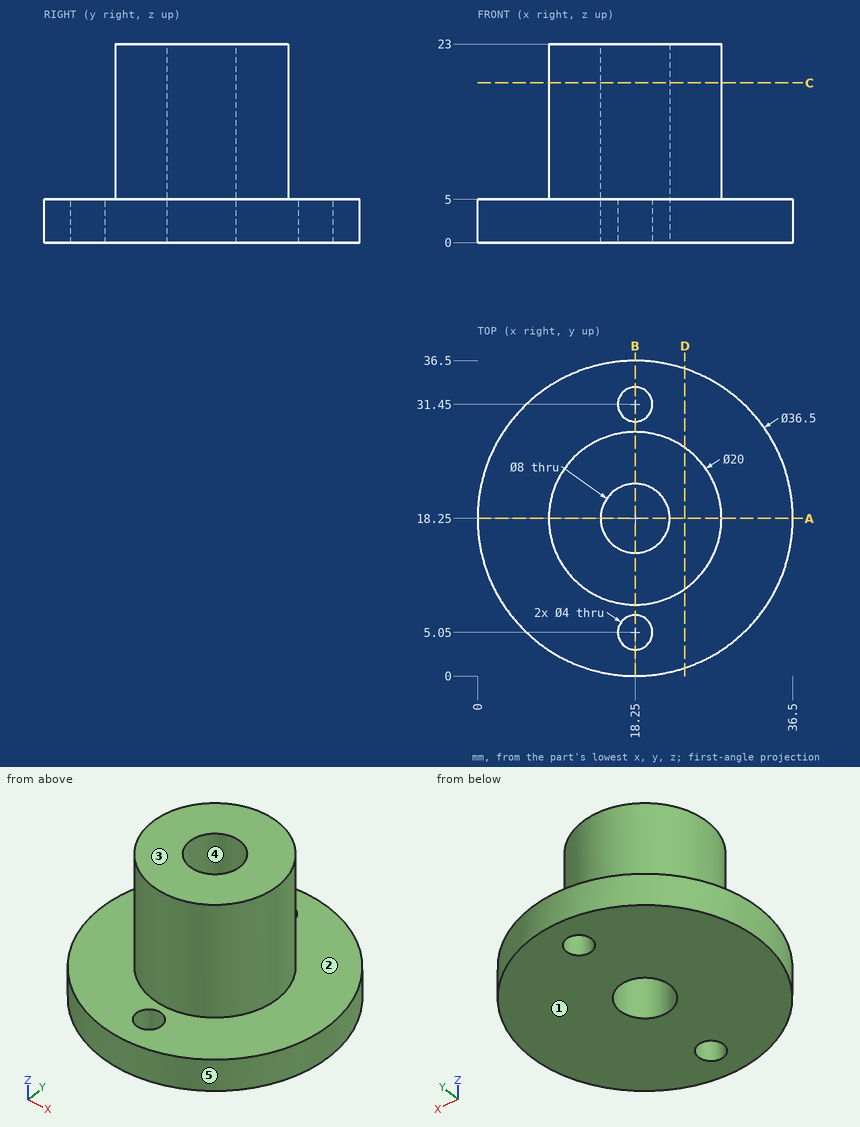
Source: three-view drawing plus pictorial views. Frame: mm from the lowest corner of the part. A direction names the side the tool comes from. Coordinates: 2 decimals unless noted, no trailing zeros. Loops run counter-clockwise (first coordinate to the right, second up) from the corner with the lowest first, then second, coordinate; pieces in that order, holes last. Notation, with made-up numbers: (42.25, 36.5) -> (55.25, 36.5) arc R13 cw to (55.25, 61.5) -> close; hole circle Ø4 at (64.5, -22.5). An arc over 180 degrees is marked (long way). Write each question's results on one line, items separated by ' | '. Start each with the question number.
Q1. Pull-direction query (X, two-part tool) for the marked faces 3, 4 and 5; classes: released by +X, released by -X, zero draft, split by the parting line, or undercut.
Q2. Pin query (flat end, axial travel): pin 1 (5 mm diameter, centred on x = 18.25, y = 5.05, fed in from -Z); pin 2 (2 mm diameter, centred on y = 6, z = 10.5, fed in from +X); pin 3 (5 mm diameter, centred on y = 6.5, z = 7, fed in from +X); pin 4 (10 mm diameter, centred on x = 28.5, z = 5.5, fed in from -Y). Return the tip coordinate at first contact, or that it passes through.
Q3. Section A-A, the plane y = 18.25. Return the cut outline in (x, z), plus the area to 4 significant figures.
Q4. Section D-D, the plane x = 24. Return the cut outline in (y, z).
Q5. Section B-B, the plane x = 18.25. Return the cut outline in (y, z).
Q6. Ray query, line 1 (Y direction, x = 18.25, z = 2.4); line 2 (Y direction, x = 18.25, z = 17); line 3 (Z direction, x = 27.5, y = 9). Return the intervals inside material, ascending. Write a range as from..to.
Q7. Reachability of the marked faces 1 and 2 from +Z, -Z, +X, -X, +Y, -Y: full face, straight path, thin tool, end or side. Return the list, or none.
Q8. Section C-C, the plane z = 18.5. Return the cut outline in (x, y), plus the area to 3 significant figures.
Found:
1) face 3: zero draft | face 4: undercut | face 5: split by the parting line
2) pin 1: z = 0 | pin 2: through | pin 3: x = 33.35 | pin 4: y = 0.78
3) outline: (0, 0) -> (14.25, 0) -> (14.25, 23) -> (8.25, 23) -> (8.25, 5) -> (0, 5) -> close; (22.25, 0) -> (36.5, 0) -> (36.5, 5) -> (28.25, 5) -> (28.25, 23) -> (22.25, 23) -> close | area: 358.5 mm2
4) outline: (0.93, 0) -> (35.57, 0) -> (35.57, 5) -> (26.43, 5) -> (26.43, 23) -> (10.07, 23) -> (10.07, 5) -> (0.93, 5) -> close
5) outline: (0, 0) -> (3.05, 0) -> (3.05, 5) -> (0, 5) -> close; (7.05, 0) -> (14.25, 0) -> (14.25, 23) -> (8.25, 23) -> (8.25, 5) -> (7.05, 5) -> close; (22.25, 0) -> (29.45, 0) -> (29.45, 5) -> (28.25, 5) -> (28.25, 23) -> (22.25, 23) -> close; (33.45, 0) -> (36.5, 0) -> (36.5, 5) -> (33.45, 5) -> close
6) line 1: 0..3.05, 7.05..14.25, 22.25..29.45, 33.45..36.5 | line 2: 8.25..14.25, 22.25..28.25 | line 3: 0..5
7) face 1: -Z, +X, -X, +Y, -Y | face 2: +Z
8) outline: circle Ø20 at (18.25, 18.25); hole circle Ø8 at (18.25, 18.25) | area: 264 mm2
